from build123d import *

# Parameters (mm, degrees)
SKETCH2_W           = 38.1
SKETCH2_H           = 38.1
SKETCH2_W_2         = 34.925
SKETCH2_H_2         = 34.925
BOSS_EXTRUDE1_DEPTH = 228.6
SKETCH3_R           = 3
CUT_EXTRUDE1_DEPTH  = 228.6


with BuildPart() as part:
    # Sketch2 → Boss-Extrude1 (new body)
    with BuildSketch(Plane(origin=(0, 0, 0), x_dir=(0, 0, -1), z_dir=(1, 0, 0))):
        with Locations((19.05, 19.05)):
            Rectangle(SKETCH2_W, SKETCH2_H)
        with Locations((19.05, 19.05)):
            Rectangle(SKETCH2_W_2, SKETCH2_H_2, mode=Mode.SUBTRACT)
    extrude(amount=BOSS_EXTRUDE1_DEPTH)

    # Sketch3 → Cut-Extrude1 (cut)
    with BuildSketch(Plane.XY):
        with Locations((25.4, 12.7)):
            Circle(SKETCH3_R)
        with Locations((152.4, 12.7)):
            Circle(SKETCH3_R)
        Polygon((0, 12.7), (25.4, 25.4), (152.4, 25.4), (177.8, 12.7), (177.8, 0), (228.6, 0), (228.6, 38.1), (0, 38.1), align=None)
    extrude(amount=-CUT_EXTRUDE1_DEPTH, mode=Mode.SUBTRACT)


solid = part.part
Verification items for the finished model (mm, model axes). A direction names the side the tool comes from. Round coordinates to 2 decimals unless told otherwise and drop trailing zeros. Write each loop counter-clockwise with the first axis right and the second up, starting at its lowest first coordinate (ties: lowest second). Pieces come first, ordered by that corner, then holes.
(1) Access from +Z, -Z, +X, -X, +Y, -Y to the whole of each face (thin tool, end or side, straight path). Record for faces 4 (the flat face through (88, 13, -1.588)), 5 (the flat face through (12.52, 18.96, -0.78)).
Returned:
face 4: +X, -X, +Y
face 5: +Z, -Z, -X, +Y
(2) Material ranges on line 1 (Y direction, x = 25.4, z = -37.6); line 2 (Z direction, x = 46, y = 17.25); line 3 (Y direction, x = 25, z = -32.5), recorded low to high.
Returned:
line 1: y = 0 to 9.7, 15.7 to 25.4
line 2: z = -38.1 to -36.51, -1.59 to 0
line 3: y = 0 to 1.59
(3) Depth check by flat-ended pin: pin 1 Ø10.5 at (x, z) = (73, -26) entering from +Y. Enter the tip coordinate at first touch or a pass-through.
Returned:
pin 1: stops at y = 1.59
(4) Mould release check, pull along Y, two halves, no side actions. Record for faces 1 (the flat face through (164.92, 19.14, -37.3)), 2 (the cylindrical face through (27.01, 15.23, -0.78)), 3 (the flat face through (88, 0, -19)): pulls with the +Y half, pulls with the -Y half, needs draft (parallel to the pull), parting line crosses it, or undercut.
Returned:
face 1: pulls with the +Y half
face 2: undercut
face 3: pulls with the -Y half
(5) Section check B-B (x = 111). Enter the section's corners in (y, z), plus the area to 3 significant figures.
Returned:
outline: (0, -38.1) - (25.4, -38.1) - (25.4, -36.51) - (1.59, -36.51) - (1.59, -1.59) - (25.4, -1.59) - (25.4, 0) - (0, 0) - close
area: 136 mm2
(6) Section check A-A (y = 23.75). Enter the section's corners in (x, z).
Returned:
outline: (22.1, -38.1) - (155.7, -38.1) - (155.7, -36.51) - (22.1, -36.51) - close; (22.1, -1.59) - (155.7, -1.59) - (155.7, 0) - (22.1, 0) - close
